Check sheet for the drawn part. Datum: minimum x, y, z corner. Units: mm. A direction names the side the tool comes from. Give positions to 0.01 mm unless a question says otherwise; leave off trailing zeros. Loops run counter-clockwise (first coordinate to the right, second up) from the corner with the lowest first, then second, coordinate; pieces in that order, holes last. Notation, with made-up numbers: (-37, 68.5) - (-20, 68.5) arc R20 cw to (-20, 102.5) - close; hole circle Ø11 at (69.5, 45.25). An arc over 180 degrees is marked (long way). Use one line per item in the form item = value.
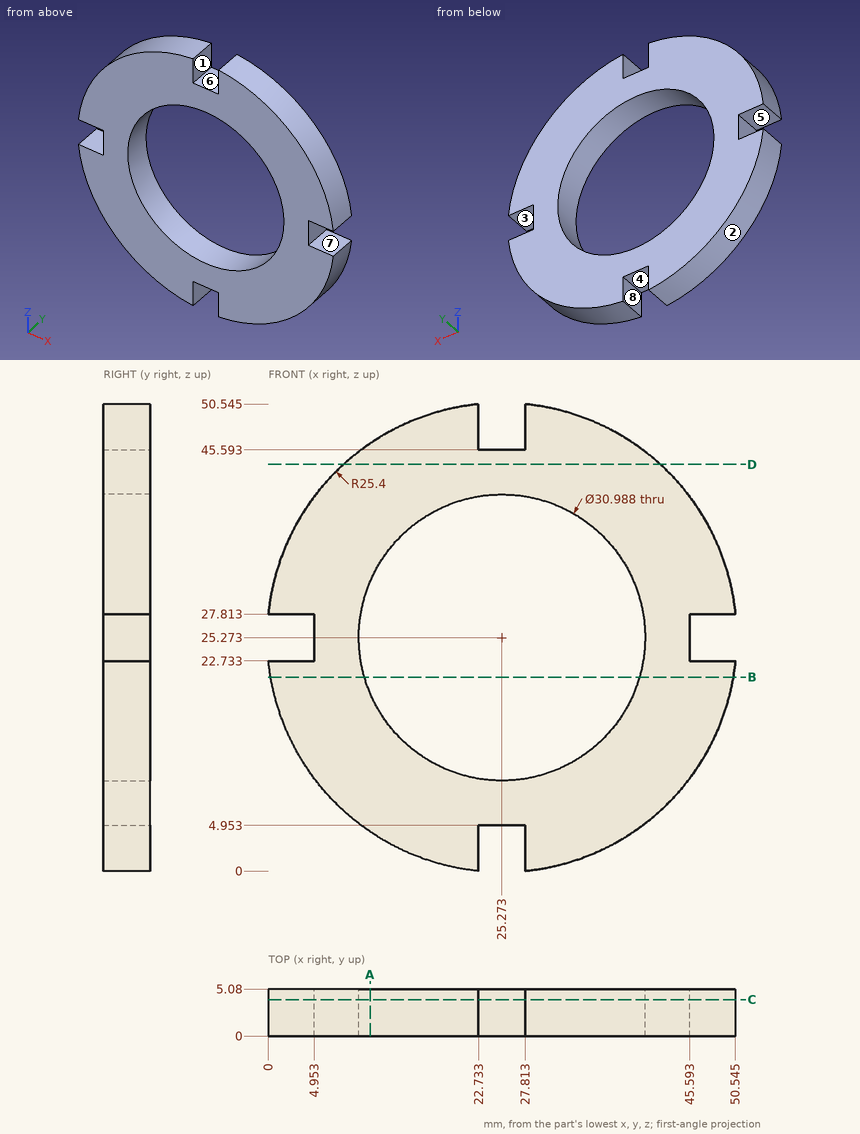
Item 1: Mould release check, pull along X, two halves, no side actions. Record for the marked faces 1, 2, 3 and 4: released by +X, released by -X, zero draft, split by the parting line, or undercut.
Answer block:
face_1 = undercut
face_2 = released by -X
face_3 = zero draft
face_4 = undercut
Item 2: Section check A-A on x = 11. Record the boundary of the cut face in (y, z).
Answer block:
outline = (0, 4.26) - (5.08, 4.26) - (5.08, 19.24) - (0, 19.24) - close; (0, 31.3) - (5.08, 31.3) - (5.08, 46.28) - (0, 46.28) - close
Item 3: Gauge pin test, flat ends, axial feed: P1, Ø1.5, axis at x = 3.5, y = 2, coming from the +Z side; P2, Ø2.5, axis at x = 25.5, y = 3.5, coming from the +Z side; P3, Ø1, axis at y = 4.5, z = 30.5, coming from the -X side. Record the tip position at first contact, or that the pin passes through.
Answer block:
P1 = 39.53
P2 = 45.59
P3 = 0.32
Item 4: Section check D-D on z = 44. Record the boundary of the cut face in (x, y), then the cut area to 3 significant figures.
Answer block:
outline = (8.11, 0) - (42.43, 0) - (42.43, 5.08) - (8.11, 5.08) - close
area = 174 mm2
Item 5: Access from +Z, -Z, +X, -X, +Y, -Y to the whole of each face (thin tool, end or side, straight path). Record for the marked faces 5, 6, 7 and 8.
Answer block:
face_5 = -X, +Y, -Y
face_6 = +Z, +Y, -Y
face_7 = +X, +Y, -Y
face_8 = -Z, +Y, -Y
Item 6: Section check B-B on z = 21. Record the boundary of the cut face in (x, y) (1 decimal).
Answer block:
outline = (0.2, 0) - (10.4, 0) - (10.4, 5.1) - (0.2, 5.1) - close; (40.2, 0) - (50.3, 0) - (50.3, 5.1) - (40.2, 5.1) - close
Item 7: Thickness scan on L1, parallel to X at y = 4.9, z = 23; L2, parallel to X at y = 4.7, z = 37.5 (1 decimal); L3, parallel to Z at x = 31.5, y = 2.2 (1 decimal). Record the ranges inside material, lowest first.
Answer block:
L1 = 4.95 to 9.95, 40.6 to 45.59
L2 = 3 to 15.8, 34.8 to 47.5
L3 = 0.6 to 11.1, 39.5 to 49.9
Item 8: Section check C-C on y = 3.95. Record the boundary of the cut face in (x, z) (1 decimal).
Answer block:
outline = (0, 22.7) arc R25.4 ccw to (22.7, 0) - (22.7, 5) - (27.8, 5) - (27.8, 0) arc R25.4 ccw to (50.5, 22.7) - (45.6, 22.7) - (45.6, 27.8) - (50.5, 27.8) arc R25.4 ccw to (27.8, 50.5) - (27.8, 45.6) - (22.7, 45.6) - (22.7, 50.5) arc R25.4 ccw to (0, 27.8) - (5, 27.8) - (5, 22.7) - close; hole circle Ø31 at (25.3, 25.3)
